```python
from build123d import *

# Parameters (mm, degrees)
BOSS_EXTRUDE1_DEPTH = 635
SKETCH2_R           = 14.2875
CUT_EXTRUDE1_DEPTH  = 26.4


with BuildPart() as part:
    # Sketch1 → Boss-Extrude1 (new body)
    with BuildSketch(Plane.XY):
        Polygon((0, 0), (0, 50.8), (25.4, 50.8), (25.4, 47.625), (3.175, 47.625), (3.175, 3.175), (25.4, 3.175), (25.4, 0), align=None)
    extrude(amount=BOSS_EXTRUDE1_DEPTH)

    # Sketch2 → Cut-Extrude1 (cut, through all)
    with BuildSketch(Plane.ZY):
        with Locations((609.6, 25.4)):
            Circle(SKETCH2_R)
    extrude(amount=-CUT_EXTRUDE1_DEPTH, mode=Mode.SUBTRACT)


solid = part.part
```
Read the model definition and answer for the solid it produces. Units are mm, in the model's axes. A direction names the side the tool comes from. Give positions to 0.01 mm unless a question says otherwise; leave off trailing zeros. Order: outer loops, then holes, each group sorted by start corner. A loop starts at its lowest first (then second) coordinate and runs counter-clockwise, first axis right, second up. Notation, with made-up numbers: (0, 74) -> (42, 74) arc R8 ccw to (42, 85) -> close; hole circle Ø2 at (56.5, 29). An arc over 180 degrees is marked (long way). One line per item, written item: value. Start each with the question number.
(1) The part is cut by section C-C (y = 18.5). Determine the outline of the cut face in (x, z) (3 decimals).
(2) The part is cut by section B-B (x = 15.75). Determine the outline of the cut face in (y, z) (3 decimals), and give its area (3 significant figures).
(3) Flat-ended cylindrical pins translate along their axes: P1, Ø1, axis at x = 3, y = 36.5, coming from the -Z side; P2, Ø2, axis at y = 38, z = 453.5, coming from the +X side (3 decimals). Find the tip coordinate at first contact, or state that the pin passes through.
(4) A tool of negligible diameter and unlimited length cuts with its end or side. For faces 1 (the flat face through (14, 3.175, 313)), 2 (the flat face through (2, 27, 0)), from which of +Z, -Z, +X, -X, +Y, -Y can it reach the whole face along a straight path? Write none if from no direction.
(5) The part is cut by section D-D (z = 167.5). Determine the outline of the cut face in (x, y) (3 decimals), and give its area (3 significant figures).
(6) For a pull along Y with two mould halves and no side action, classify faces 3 (the flat face through (13, 0, 313)), 4 (the flat face through (2, 27, 635)), 5 (the flat face through (14, 47.625, 313)) as released by +Y, released by -Y, zero draft, split by the parting line, or undercut.
(7) The part is cut by section A-A (z = 609.6). Determine the outline of the cut face in (x, y) (1 decimal), and give its area (3 significant figures).
(8) Straight lines are drawn through the part: L1, parallel to Y at x = 12, z = 597.5 (3 decimals); L2, parallel to Y at x = 2.05, z = 609.6; L3, parallel to X at y = 19, z = 164.5 (3 decimals). For each, find the intervals that lie inside material, in ascending order.
Taken from the geometry:
1. outline: (0, 0) -> (3.175, 0) -> (3.175, 597.089) -> (0, 597.089) -> close; (0, 622.111) -> (3.175, 622.111) -> (3.175, 635) -> (0, 635) -> close
2. outline: (0, 0) -> (3.175, 0) -> (3.175, 635) -> (0, 635) -> close; (47.625, 0) -> (50.8, 0) -> (50.8, 635) -> (47.625, 635) -> close
2. area: 4,030 mm^2
3. P1: z = 0
3. P2: x = 3.175
4. face 1: +Z, -Z, +X
4. face 2: -Z, +X, -X, +Y, -Y
5. outline: (0, 0) -> (25.4, 0) -> (25.4, 3.175) -> (3.175, 3.175) -> (3.175, 47.625) -> (25.4, 47.625) -> (25.4, 50.8) -> (0, 50.8) -> close
5. area: 302 mm^2
6. face 3: released by -Y
6. face 4: zero draft
6. face 5: undercut
7. outline: (0, 0) -> (25.4, 0) -> (25.4, 3.2) -> (3.2, 3.2) -> (3.2, 11.1) -> (0, 11.1) -> close; (0, 39.7) -> (3.2, 39.7) -> (3.2, 47.6) -> (25.4, 47.6) -> (25.4, 50.8) -> (0, 50.8) -> close
7. area: 212 mm^2
8. L1: 0 to 3.175, 47.625 to 50.8
8. L2: 0 to 11.11, 39.69 to 50.8
8. L3: 0 to 3.175
